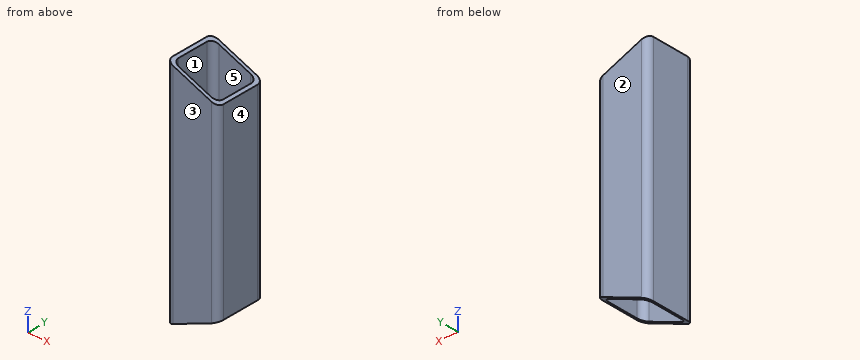
```python
from build123d import *

# Parameters (mm, degrees)
F1_W     = 25.4
F1_H     = 25.4
F2_DEPTH = 114.3
F4_DEPTH = 25.4
F5_R     = 3.175


# Not quite as in the source:
# - a variable given as a bare number and used for a length is read in inches; the dataset says mm whatever the document's units were


with BuildPart() as f2:
    # F1 (on Top) → F2 (new body)
    with BuildSketch(Plane.XY):
        Rectangle(F1_W, F1_H)
        with BuildLine():
            ThreePointArc((-11.049, 7.874), (-10.1190640303, 10.1190640303), (-7.874, 11.049))
            Line((-7.874, 11.049), (7.874, 11.049))
            ThreePointArc((7.874, 11.049), (10.1190640303, 10.1190640303), (11.049, 7.874))
            Line((11.049, 7.874), (11.049, -7.874))
            ThreePointArc((11.049, -7.874), (10.1190640303, -10.1190640303), (7.874, -11.049))
            Line((7.874, -11.049), (-7.874, -11.049))
            ThreePointArc((-7.874, -11.049), (-10.1190640303, -10.1190640303), (-11.049, -7.874))
            Line((-11.049, -7.874), (-11.049, 7.874))
        make_face(mode=Mode.SUBTRACT)
    extrude(amount=F2_DEPTH)

    # F3 (on face) → F4 (cut)
    with BuildSketch(Plane.XZ.offset(12.7)):
        Polygon((12.7, 10.5210244843), (-12.7, 0), (12.7, 0), align=None)
        Polygon((12.7, 114.3), (-12.7, 114.3), (12.7, 103.7789755157), align=None)
    extrude(amount=-F4_DEPTH, mode=Mode.SUBTRACT)

    # F5
    f5_edges = [f2.edges().sort_by_distance(p)[0] for p in [
        (-12.7, 12.7, 57.15),
        (12.7, 12.7, 57.15),
        (-12.7, -12.7, 57.15),
        (12.7, -12.7, 57.15),
    ]]
    fillet(f5_edges, radius=F5_R)


solid = f2.part
```
Geometry: final body of the model. Coordinates: model frame, mm. Face numbers are marked on the shaded views. A direction names the side the tool comes from. Round coordinates to 2 decimals unless told otherwise and drop trailing zeros. Order: outer loops, then holes, each group sorted by start corner. A loop starts at its lowest first (then second) coordinate and runs counter-clockwise, first axis right, second up. Notation, with made-up numbers: (78.5, 3) - (85.5, 3) arc R19 ccw to (85.5, 8) - close; hole circle Ø1 at (66.5, 8). An arc over 180 degrees is marked (long way). Write item = value, one per line. Start each with the question number.
Q1. Cut plane A-A on z = 94. Return the cut outline in (x, y) (3 decimals).
Q2. Pull-direction query (Y, two-part tool) for the marked faces 3, 4 and 5; classes: +Y half, -Y half, draft (parallel to the pull), parting line (faces both ways), or undercut.
Q3. Access query for the marked faces 1 and 2. Directions: +Z, -Z, +X, -X, +Y, -Y. A direction counts if a zero-diameter tool reaches every point of the face in a straight line with its end or side. Return the directions, or none.
Q4. Ray query, line 1 (Y direction, x = 3.5, z = 93); line 2 (Y direction, x = 10.75, z = 11.5). Return the intervals inside material, ascending. Write a range as from..to.
Q5. Cut plane B-B on y = 6. Return the cut outline in (x, z).
Q6. Pin query (flat end, axial travel): pin 1 (1.5 mm diameter, centred on x = -10, y = 8, fed in from -Z). Return the tip coordinate at first contact, or that it passes through.
Q7. Cut plane C-C on x = 0.25. Return the cut outline in (y, z).
Outcome:
q1.outline = (-12.7, -9.525) arc R3.175 ccw to (-9.525, -12.7) - (9.525, -12.7) arc R3.175 ccw to (12.7, -9.525) - (12.7, 9.525) arc R3.175 ccw to (9.525, 12.7) - (-9.525, 12.7) arc R3.175 ccw to (-12.7, 9.525) - close; hole (-11.049, -7.874) arc R3.175 ccw to (-7.874, -11.049) - (7.874, -11.049) arc R3.175 ccw to (11.049, -7.874) - (11.049, 7.874) arc R3.175 ccw to (7.874, 11.049) - (-7.874, 11.049) arc R3.175 ccw to (-11.049, 7.874) - close
q2.face_3 = -Y half
q2.face_4 = draft
q2.face_5 = undercut
q3.face_1 = +Z, -Z
q3.face_2 = +Z, -Z, +X, -X, +Y
q4.line_1 = -12.7..-11.05, 11.05..12.7
q4.line_2 = -12.45..-9.22, 9.22..12.45
q5.outline = (-12.7, 0) - (-11.05, 0.68) - (-11.05, 113.62) - (-12.7, 114.3) - close; (11.05, 9.84) - (12.7, 10.52) - (12.7, 103.78) - (11.05, 104.46) - close
q6.pin_1 = through
q7.outline = (-12.7, 5.36) - (-11.05, 5.36) - (-11.05, 108.94) - (-12.7, 108.94) - close; (11.05, 5.36) - (12.7, 5.36) - (12.7, 108.94) - (11.05, 108.94) - close
